Geometry: final body of the model. Coordinates: model frame, mm. Round coordinates to 2 decimals unless told otherwise and drop trailing zeros. Write each loop counter-clockwise with the first axis right and the second up, starting at its lowest first coordinate (ties: lowest second). Pieces come first, ordered by that corner, then holes. Notation, with made-up numbers: M -38.5,22 L 5.5,22 A30 ccw 5.5,61 Z; hole C 24,53.5 d6. An arc over 180 degrees is marked long. Put each result on its own line as item: value. Start each with the question number.
```python
from build123d import *

# Parameters (mm, degrees)
F0_W     = 38.1
F0_H     = 890.5875
F1_DEPTH = 19.05
F3_DEPTH = 19.051
F4_R     = 3.175


with BuildPart() as f1:
    # F0 (on Front) → F1 (new body)
    with BuildSketch(Plane.XZ):
        Rectangle(F0_W, F0_H)
    extrude(amount=F1_DEPTH)

    # F2 (on face) → F3 (cut, through all)
    with BuildSketch(Plane.XZ.offset(19.05)):
        Polygon((19.05, 445.29375), (-19.05, 445.29375), (19.05, 407.19375), align=None)
    extrude(amount=-F3_DEPTH, mode=Mode.SUBTRACT)

    # F4
    f4_edges = [f1.edges().sort_by_distance(p)[0] for p in [
        (-19.05, -19.05, 0),
        (19.05, -19.05, -19.05),
    ]]
    fillet(f4_edges, radius=F4_R)


solid = f1.part
```
1) First-contact query: pin 1 (4 mm diameter, centred on x = -10.5, z = -13.5, fed in from +Y); pin 2 (5 mm diameter, centred on x = -2.5, y = -10, fed in from +Z); pin 3 (1 mm diameter, centred on x = -0.5, y = -5, fed in from +Z); pin 4 (2 mm diameter, centred on x = 5.5, y = -14.5, fed in from +Z). Flat tips, straight axial feed; report the tip coordinate or a pass-through.
2) Section B-B, the plane x = 1. Output: boundary loops of the cut face in (y, z).
3) Section A-A, the plane y = -8.75. Output: boundary loops of the cut face in (x, z).
4) Ray query, probe 1 along Y at (x, z) = (16, -288.5); probe 2 along Z at (x, y) = (2.5, -12); probe 3 along Z at (x, y) = (4.5, -0.75). Return the intervals inside material, ascending.
Solved:
1. pin 1: stops at y = 0
1. pin 2: stops at z = 431.24
1. pin 3: stops at z = 427.24
1. pin 4: stops at z = 421.74
2. outline: M -19.05,-445.29 L 0,-445.29 L 0,425.24 L -19.05,425.24 Z
3. outline: M -19.05,-445.29 L 19.05,-445.29 L 19.05,407.19 L -19.05,445.29 Z
4. probe 1: y = -19.05 to 0
4. probe 2: z = -445.29 to 423.74
4. probe 3: z = -445.29 to 421.74
